Part model, mm, in its own coordinate system. Face numbers are marked on the shaded views. Round coordinates to 2 decimals unless told otherwise and drop trailing zeros. Order: outer loops, then holes, each group sorted by start corner. A loop starts at its lowest first (then second) coordinate and runs counter-clockwise, first axis right, second up. Notation, with made-up numbers: (-8, 7.25) -> (31, 7.25) arc R15 cw to (31, 23.25) -> close; hole circle Ø1 at (37.25, 26.5). An arc over 180 degrees is marked (long way). Use CSV: the item, a comma, the result in double quotes.
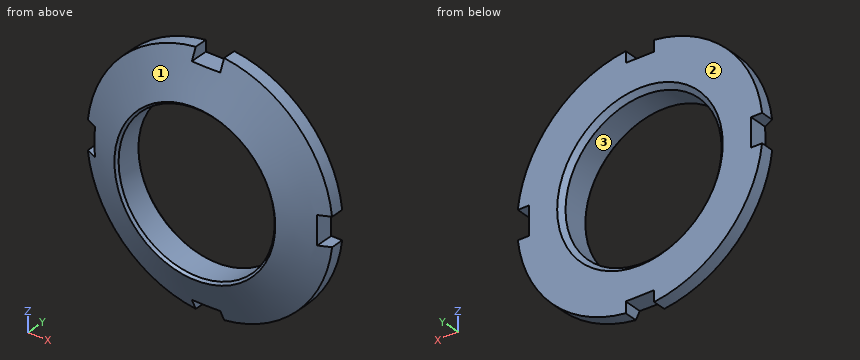
Autodesk Inventor part; units mm, degrees
ref_plane "YZ Plane" through (0, 0, 0) normal (1, 0, 0) x (0, 1, 0)
ref_plane "XZ Plane" through (0, 0, 0) normal (0, 1, 0) x (-1, 0, 0)
ref_plane "XY Plane" through (0, 0, 0) normal (0, 0, 1) x (1, 0, 0)
sketch "Эскиз1" plane through (0, 0, 0) normal (0, 0, 1) x (1, 0, 0)
  line L0 (0, 3.5) -> (0, -3.5)
  line L1 (17, -3.5) -> (26, 0.6968)
  line L2 (26, 0.6968) -> (26, 3.5)
  line L3 (26, 3.5) -> (17.5, 3.5)
  line L4 (17, -3.5) -> (16.5, -3)
  line L5 (16.5, -3) -> (16.5, 2.5)
  line L6 (0, -3.5) -> (17, -3.5) construction
  line L7 (16.5, 2.5) -> (17.5, 3.5)
  point P0 (0, 0)
  point P1 (0, 0)
  point P2 (16.5, 3.5)
  dimension "d0" = 7
  dimension "d1" = 34
  dimension "d2" = 33
  dimension "d3" = 25
  dimension "d4" = 52
  dimension "d5" = 45
  dimension "d6" = 1
  dimension "d7" = 45
revolve "Вращение1" add sketch "Эскиз1" angle 360 about axis through (0, 3.5, 0) along (0, -1, 0)
sketch "Эскиз2" plane through (0, 3.5, 0) normal (0, 1, 0) x (1, 0, 0)
  line L0 (-3, 26) -> (3, 26)
  line L1 (3, 26) -> (3, 23.5)
  line L2 (3, 23.5) -> (-3, 23.5)
  line L3 (-3, 23.5) -> (-3, 26)
  circle A0 centre (0, 0) radius 26
  point P0 (0, 0)
  point P1 (0, 23.5)
  point P2 (3, 25.8263)
  point P3 (-3, 25.8263)
  dimension "d9" = 6
  dimension "d10" = 2.5
extrude "Выдавливание1" cut sketch "Эскиз2" against normal through all contours A0 L1 L2 L3 picked at (0, 24.3333)
pattern_circular "Круговой массив1" count 4 over 360 about axis through (0, 2.0984, 0) along (0, -1, 0) of "Выдавливание1"
thread "Резьба1"
properties part number "75. Гайка промежуточного вала"
(1) Cut at A-A, the plane x = 0. Give the cut face in (y, z).
Reply:
outline,"(-3.5, -17) -> (-0.47, -23.5) -> (3.5, -23.5) -> (3.5, -17.5) -> (2.5, -16.5) -> (-3, -16.5) -> close; (-3.5, 17) -> (-3, 16.5) -> (2.5, 16.5) -> (3.5, 17.5) -> (3.5, 23.5) -> (-0.47, 23.5) -> close"
(2) Cut at B-B, the plane z = 0. Give the cut face in (x, y).
Reply:
outline,"(-23.5, -0.47) -> (-17, -3.5) -> (-16.5, -3) -> (-16.5, 2.5) -> (-17.5, 3.5) -> (-23.5, 3.5) -> close; (16.5, -3) -> (17, -3.5) -> (23.5, -0.47) -> (23.5, 3.5) -> (17.5, 3.5) -> (16.5, 2.5) -> close"
(3) Probe probe 1 along Z at (x, y) = (0, 0.2); probe 2 along X at (y, z) = (1, -10.5); probe 3 along Z at (x, y) = (8.5, -0.25). List the from-to ranges inside material, lowest first. Write a range as [from, to].
Reply:
probe 1,"[-23.5, -16.5], [16.5, 23.5]"
probe 2,"[-23.79, -12.73], [12.73, 23.79]"
probe 3,"[-22.41, -14.14], [14.14, 22.41]"
(4) Drop flat-ended pins along their axis: P1, Ø1.2, axis at y = 1, z = 1, coming from the -X side; P2, Ø1.2, axis at x = 1, y = 2, coming from the +Z side; P3, Ø2.5, axis at y = 2, z = 25, coming from the +X side. Give the stop position or say it passes through.
Reply:
P1,"x = -23.5"
P2,"z = 23.5"
P3,"x = 10.58"
(5) Pull direction X, two halves, no side cores. Call the marked faces 1, 2 and 3: released by +X, released by -X, zero draft, split by the parting line, or undercut.
Reply:
face 1,"split by the parting line"
face 2,"zero draft"
face 3,"undercut"
